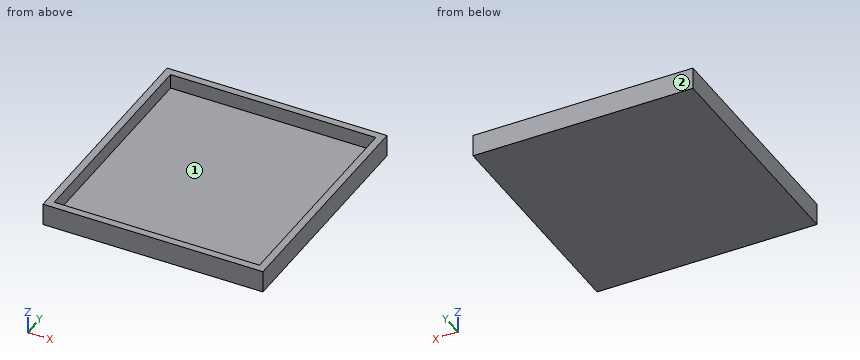
```python
from build123d import *

# Parameters (mm, degrees)
SKETCH1_W           = 150
SKETCH1_H           = 160
BOSS_EXTRUDE1_DEPTH = 5
SKETCH2_W           = 150
SKETCH2_H           = 5
BOSS_EXTRUDE2_DEPTH = 10
SKETCH3_W           = 5
SKETCH3_H           = 155
BOSS_EXTRUDE3_DEPTH = 10
SKETCH4_W           = 145
SKETCH4_H           = 5
BOSS_EXTRUDE4_DEPTH = 10
SKETCH5_W           = 5
SKETCH5_H           = 150
BOSS_EXTRUDE5_DEPTH = 10


with BuildPart() as part:
    # Sketch1 → Boss-Extrude1 (new body)
    with BuildSketch(Plane.XY):
        with Locations((75, 80)):
            Rectangle(SKETCH1_W, SKETCH1_H)
    extrude(amount=-BOSS_EXTRUDE1_DEPTH)

    # Sketch2 → Boss-Extrude2 (add)
    with BuildSketch(Plane.XY):
        with Locations((75, 157.5)):
            Rectangle(SKETCH2_W, SKETCH2_H)
    extrude(amount=BOSS_EXTRUDE2_DEPTH)

    # Sketch3 → Boss-Extrude3 (add)
    with BuildSketch(Plane.XY):
        with Locations((147.5, 77.5)):
            Rectangle(SKETCH3_W, SKETCH3_H)
    extrude(amount=BOSS_EXTRUDE3_DEPTH)

    # Sketch4 → Boss-Extrude4 (add)
    with BuildSketch(Plane.XY):
        with Locations((72.5, 2.5)):
            Rectangle(SKETCH4_W, SKETCH4_H)
    extrude(amount=BOSS_EXTRUDE4_DEPTH)

    # Sketch5 → Boss-Extrude5 (add)
    with BuildSketch(Plane.XY):
        with Locations((2.5, 80)):
            Rectangle(SKETCH5_W, SKETCH5_H)
    extrude(amount=BOSS_EXTRUDE5_DEPTH)


solid = part.part
```
For this review, take the finished solid that the model builds, in its own axes (mm). Face numbers are marked on the shaded views. Give positions to 0.01 mm unless a question says otherwise; leave off trailing zeros. Write each loop counter-clockwise with the first axis right and the second up, starting at its lowest first coordinate (ties: lowest second). Pieces come first, ordered by that corner, then holes. Notation, with made-up numbers: M 43,-20 L 55,-20 A17 ccw 55,-16 Z; hole C -10.5,-18 d8. An arc over 180 degrees is marked long. One line per item, written item: value.
1) For P1, Ø3, axis at x = 43.5, z = 6.5, coming from the -Y side; P2, Ø12, axis at x = 124.5, y = 77.5, coming from the +Z side, all flat-tipped, find the tip position at first contact; note any pin that passes through.
Results are:
P1: stops at y = 0
P2: stops at z = 0
2) Take a section at B-B, the plane z = 4.5. Write out the cut boundary in (x, y), then the cut area to 3 significant figures.
Results are:
outline: M 0,0 L 150,0 L 150,160 L 0,160 Z; hole M 5,5 L 145,5 L 145,155 L 5,155 Z
area: 3,000 mm²
3) Take a section at A-A, the plane x = 104. Write out the cut boundary in (y, z), then the cut area to 3 significant figures.
Results are:
outline: M 0,-5 L 160,-5 L 160,10 L 155,10 L 155,0 L 5,0 L 5,10 L 0,10 Z
area: 900 mm²
4) The part is to be moulded in two halves that separate along X. For the marked faces 1 and 2, say which applies: +X half, -X half, draft (parallel to the pull), parting line (faces both ways), or undercut.
Results are:
face 1: undercut
face 2: draft
5) For line 1 (X direction, y = 129, z = 2.5); line 2 (Y direction, x = 111.5, z = 8.5); line 3 (Z direction, x = 61, y = 16), list the stretches that pass through material, from the lowest coordinate up. Write a range as from..to.
Results are:
line 1: x = 0..5, 145..150
line 2: y = 0..5, 155..160
line 3: z = -5..0
6) Take a section at C-C, the plane y = 141.5. Write out the cut boundary in (x, z), then the cut area to 3 significant figures.
Results are:
outline: M 0,-5 L 150,-5 L 150,10 L 145,10 L 145,0 L 5,0 L 5,10 L 0,10 Z
area: 850 mm²
